CAD build for the part. Positions are in the model's coordinates, mm. A direction names the side the tool comes from. Coordinates: 2 decimals unless noted, no trailing zeros. Order: outer loops, then holes, each group sorted by start corner. A loop starts at its lowest first (then second) coordinate and runs counter-clockwise, first axis right, second up. Notation, with made-up numbers: (81.25, -12.75) - (137.25, -12.75) arc R8 ccw to (137.25, -0.75) - close; hole circle Ø6 at (0, 60.5). An arc over 180 degrees is marked (long way). Use one line per item in the form item = value.
```python
from build123d import *

# Parameters (mm, degrees)
SKETCH1_W                                        = 47.06874
SKETCH1_H                                        = 16.933333333
CBORE_FOR_1_4_SOCKET_HEAD_CAP_SCREW1_D           = 6.7564
CBORE_FOR_1_4_SOCKET_HEAD_CAP_SCREW1_CBORE_D     = 11.1125
CBORE_FOR_1_4_SOCKET_HEAD_CAP_SCREW1_CBORE_DEPTH = 6.35
F_3_16_0_1875_DOWEL_HOLE1_D                      = 4.7625
F_3_16_0_1875_DOWEL_HOLE1_DEPTH                  = 9.652
F_3_16_0_1875_DOWEL_HOLE1_TIP                    = 1.430799349


with BuildPart() as part:
    # Sketch1 → Revolve1 (revolve)
    with BuildSketch(Plane.XY, mode=Mode.PRIVATE) as revolve1_sk:
        with Locations((23.53437, 29.633333334)):
            Rectangle(SKETCH1_W, SKETCH1_H)
    revolve(revolve1_sk.sketch.rotate(Axis((0, 0, 0), (1, 0, 0)), 90), axis=Axis((0, 0, 0), (1, 0, 0)))

    # CBORE for 1/4 Socket Head Cap Screw1 (through all)
    with Locations(Plane.ZY):
        with Locations((0, 29.633333333), (20.953930949, 20.953930949), (29.633333333, 0), (20.953930949, -20.953930949), (0, -29.633333333), (-20.953930949, -20.953930949), (-29.633333333, 0), (-20.953930949, 20.953930949)):
            CounterBoreHole(CBORE_FOR_1_4_SOCKET_HEAD_CAP_SCREW1_D / 2, CBORE_FOR_1_4_SOCKET_HEAD_CAP_SCREW1_CBORE_D / 2, CBORE_FOR_1_4_SOCKET_HEAD_CAP_SCREW1_CBORE_DEPTH)

    # 3/16 (0.1875) Dowel Hole1
    with Locations(Plane.ZY):
        with Locations((-11.542689029, 27.866516399), (27.866516399, 11.542689029), (11.542689029, -27.866516399), (-27.866516399, -11.542689029)):
            Hole(F_3_16_0_1875_DOWEL_HOLE1_D / 2, depth=F_3_16_0_1875_DOWEL_HOLE1_DEPTH)
            with Locations((0, 0, -(F_3_16_0_1875_DOWEL_HOLE1_DEPTH + F_3_16_0_1875_DOWEL_HOLE1_TIP / 2))):  # 118° drill point
                Cone(0, F_3_16_0_1875_DOWEL_HOLE1_D / 2, F_3_16_0_1875_DOWEL_HOLE1_TIP, mode=Mode.SUBTRACT)


solid = part.part
```
Item 1: Drill centre lines: line 1 (Y direction, x = 38, z = 0); line 2 (Y direction, x = 3, z = -12); line 3 (Y direction, x = 20.5, z = 5). Where is each one in solid material? Low to high. Write a range as [from, to].
Derived:
line_1 = [-38.1, -33.01], [-26.26, -21.17], [21.17, 26.26], [33.01, 38.1]
line_2 = [-36.16, -17.44], [17.44, 25.53], [30.2, 36.16]
line_3 = [-37.77, -20.57], [20.57, 37.77]
Item 2: Cut at A-A, the plane y = 0. Write the cut outline in (x, z).
Derived:
outline = (0, -38.1) - (47.07, -38.1) - (47.07, -33.01) - (6.35, -33.01) - (6.35, -35.19) - (0, -35.19) - close; (0, -24.08) - (6.35, -24.08) - (6.35, -26.26) - (47.07, -26.26) - (47.07, -21.17) - (0, -21.17) - close; (0, 21.17) - (47.07, 21.17) - (47.07, 26.26) - (6.35, 26.26) - (6.35, 24.08) - (0, 24.08) - close; (0, 35.19) - (6.35, 35.19) - (6.35, 33.01) - (47.07, 33.01) - (47.07, 38.1) - (0, 38.1) - close
Item 3: 3-axis set-ups, long thin cutter, end or side, ignore diameter. For faces 1 (the face through (4.894, 28.582, -13.814)), 2 (the face through (26.99, -24.25, 21.69)): which of +Z, -Z, +X, -X, +Y, -Y reach the whole face in a straight line?
Derived:
face_1 = -X
face_2 = +X, -X
Item 4: Two-plate mould, pull along Y, no slides. Class faces 3 (the face through (6.35, -30, 4)), 4 (the face through (23.864, -20.987, -2.755)), 5 (the face through (0, 16, -16)): +Y half, -Y half, draft (parallel to the pull), parting line (faces both ways), or undercut.
Derived:
face_3 = undercut
face_4 = undercut
face_5 = draft
Item 5: Drop flat-ended pins along their axis: pin 1 (10 mm diameter, centred on y = -20.95, z = 20.95, fed in from -X); pin 2 (1 mm diameter, centred on x = 42, z = 15, fed in from +Y); pin 3 (1 mm diameter, centred on x = 28, z = 13.5, fed in from -Y). Give the stop position or say it passes through.
Derived:
pin_1 = 6.35
pin_2 = 35.23
pin_3 = -35.81
